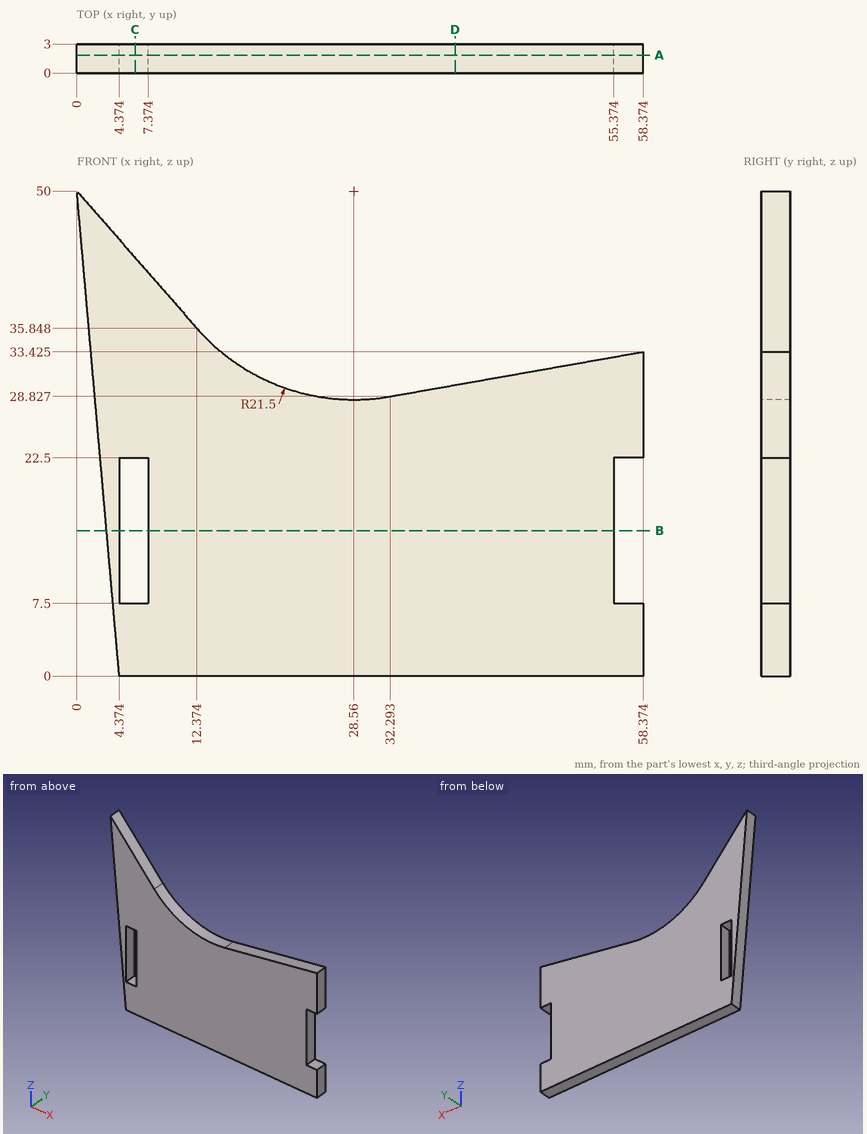
Could you check a few things on this drawing? It's one solid part, dimensions in mm from its lowest x, y, z. Coordinates: 2 decimals unless noted, no trailing zeros. Write each loop counter-clockwise with the first axis right and the second up, starting at its lowest first coordinate (ties: lowest second). Pieces come first, ordered by that corner, then holes. Notation, with made-up numbers: (73.5, -5) - (132.5, -5) arc R20 ccw to (132.5, 8) - close; hole circle Ø3 at (45, 36). An arc over 180 degrees is marked (long way). Return JSON: item names as keys, results as strings. Group by question number.
Item 1: If we section it at A-A (y = 1.85): Write out the boundary of the cut face in (x, z) (1 decimal), then the cut area to 3 significant figures.
Item 2: Please list where these lines run through material, in increasing order: probe 1 along X at (y, z) = (1.1, 16.5) (1 decimal); probe 2 along X at (y, z) = (1.9, 16) (1 decimal); probe 3 along Z at (x, y) = (11, 0.65).
Item 3: If we section it at C-C (x = 6): Write out the boundary of the cut face in (y, z).
Item 4: I'm going to push flat-ended pins straight in: pin 1 Ø1.5 at (x, y) = (6.5, 2) entering from +Z (1 decimal); pin 2 Ø1.5 at (y, z) = (2, 13.5) entering from +X; pin 3 Ø1.5 at (x, y) = (57, 1.5) entering from +Z (1 decimal). Where does each tip first touch, or does it pass through?
Item 5: If we section it at B-B (z = 15): Write out the boundary of the cut face in (x, y) (1 decimal).
Item 6: If we section it at D-D (x = 39): Write out the boundary of the cut face in (y, z).
Return value:
{
 "1": {"outline": "(0, 50) - (4.4, 0) - (58.4, 0) - (58.4, 7.5) - (55.4, 7.5) - (55.4, 22.5) - (58.4, 22.5) - (58.4, 33.4) - (32.3, 28.8) arc R21.5 cw to (12.4, 35.8) - close; hole (4.4, 7.5) - (7.4, 7.5) - (7.4, 22.5) - (4.4, 22.5) - close", "area": "1,750 mm^2"},
 "2": {"probe 1": "x = 2.9 to 4.4, 7.4 to 55.4", "probe 2": "x = 3 to 4.4, 7.4 to 55.4", "probe 3": "z = 0 to 37.42"},
 "3": {"outline": "(0, 0) - (3, 0) - (3, 7.5) - (0, 7.5) - close; (0, 22.5) - (3, 22.5) - (3, 43.14) - (0, 43.14) - close"},
 "4": {"pin 1": "stops at z = 43.4", "pin 2": "stops at x = 55.37", "pin 3": "stops at z = 33.3"},
 "5": {"outline": "(3.1, 0) - (4.4, 0) - (4.4, 3) - (3.1, 3) - close; (7.4, 0) - (55.4, 0) - (55.4, 3) - (7.4, 3) - close"},
 "6": {"outline": "(0, 0) - (3, 0) - (3, 30.01) - (0, 30.01) - close"}
}
